Autodesk Inventor part; units mm, degrees
ref_plane "Work Plane1" through (-4.5785, -14.9902, 9) normal (0, 0, -1) x (0, 1, 0)
ref_plane "YZ Plane" through (0, 0, 0) normal (1, 0, 0) x (0, 1, 0)
ref_plane "XZ Plane" through (0, 0, 0) normal (0, 1, 0) x (-1, 0, 0)
sketch "Sketch1" plane through (0, 0, 0) normal (0, 0, 1) x (1, 0, 0)
  arc A0 (-8.6401, -8.1682) -> (6.2316, -10.1261) centre (-1.5676, -11.9073) ccw
  line L0 (7.4345, -0.9889) -> (6.2316, -10.1261)
  line L1 (-7.4371, 0.969) -> (7.4345, -0.9889)
  line L2 (-8.6401, -8.1682) -> (-7.4371, 0.969)
  line L3 (0.03, -17.852) -> (-0.1568, -19.2714)
  line L4 (-0.1568, -19.2714) -> (-0.6894, -19.2013)
  spline S0 degree 3 poles (-0.6894, -19.2013) (-0.7386, -19.1939) (-0.8276, -19.1805) (-0.9085, -19.1413) (-0.9446, -19.1238) knots 0 0 0 0 0.014823 0.02681 0.02681 0.02681 0.02681
  spline S1 degree 3 poles (-0.9446, -19.1238) (-0.9734, -19.1035) (-1.0308, -19.0631) (-1.0644, -19.0015) (-1.0811, -18.9709) knots 0 0 0 0 0.010419 0.020741 0.020741 0.020741 0.020741
  spline S2 degree 3 poles (-1.0811, -18.9709) (-1.0934, -18.9389) (-1.1175, -18.8762) (-1.1139, -18.8091) (-1.1121, -18.7762) knots 0 0 0 0 0.010155 0.019912 0.019912 0.019912 0.019912
  spline S3 degree 3 poles (-1.1121, -18.7762) (-1.106, -18.7465) (-1.0937, -18.6864) (-1.0581, -18.6365) (-1.0402, -18.6114) knots 0 0 0 0 0.008998 0.018167 0.018167 0.018167 0.018167
  spline S4 degree 3 poles (-1.0402, -18.6114) (-1.0175, -18.5881) (-0.9702, -18.5394) (-0.907, -18.5143) (-0.874, -18.5012) knots 0 0 0 0 0.009628 0.020138 0.020138 0.020138 0.020138
  spline S5 degree 3 poles (-0.874, -18.5012) (-0.912, -18.4819) (-0.9849, -18.4448) (-1.0323, -18.3782) (-1.055, -18.3464) knots 0 0 0 0 0.012589 0.024139 0.024139 0.024139 0.024139
  spline S6 degree 3 poles (-1.055, -18.3464) (-1.071, -18.3116) (-1.1036, -18.2405) (-1.0985, -18.1623) (-1.096, -18.1224) knots 0 0 0 0 0.011297 0.023097 0.023097 0.023097 0.023097
  spline S7 degree 3 poles (-1.096, -18.1224) (-1.09, -18.0901) (-1.0782, -18.0263) (-1.0456, -17.9702) (-1.0294, -17.9425) knots 0 0 0 0 0.009763 0.019307 0.019307 0.019307 0.019307
  spline S8 degree 3 poles (-1.0294, -17.9425) (-1.0117, -17.9179) (-0.9781, -17.8713) (-0.9305, -17.8392) (-0.9079, -17.824) knots 0 0 0 0 0.009007 0.017087 0.017087 0.017087 0.017087
  spline S9 degree 3 poles (-0.9079, -17.824) (-0.8832, -17.8123) (-0.8309, -17.7874) (-0.7736, -17.7788) (-0.7433, -17.7743) knots 0 0 0 0 0.008157 0.017283 0.017283 0.017283 0.017283
  spline S10 degree 3 poles (-0.7433, -17.7743) (-0.7078, -17.7719) (-0.6303, -17.7668) (-0.5531, -17.7758) (-0.5112, -17.7807) knots 0 0 0 0 0.010638 0.023262 0.023262 0.023262 0.023262
  line L5 (-0.5112, -17.7807) -> (0.03, -17.852)
  line L6 (-3.4981, -17.3875) -> (-3.685, -18.8069)
  line L7 (-3.685, -18.8069) -> (-3.8728, -18.7821)
  line L8 (-3.8728, -18.7821) -> (-3.7802, -18.0783)
  line L9 (-3.7802, -18.0783) -> (-4.5777, -18.6893)
  line L10 (-4.5777, -18.6893) -> (-4.8323, -18.6558)
  line L11 (-4.8323, -18.6558) -> (-4.1612, -18.1591)
  line L12 (-4.1612, -18.1591) -> (-4.6716, -17.233)
  line L13 (-4.6716, -17.233) -> (-4.4237, -17.2656)
  line L14 (-4.4237, -17.2656) -> (-4.0129, -18.0506)
  line L15 (-4.0129, -18.0506) -> (-3.7507, -17.8546)
  line L16 (-3.7507, -17.8546) -> (-3.686, -17.3627)
  line L17 (-3.686, -17.3627) -> (-3.4981, -17.3875)
  circle A1 centre (-5.3501, -2.3316) radius 1.25
  circle A2 centre (-0.3929, -2.9842) radius 1.25
  circle A3 centre (4.5643, -3.6369) radius 1.25
  line L18 (-1.8861, -17.5997) -> (-1.7118, -17.6227)
  line L19 (-1.7118, -17.6227) -> (-1.858, -18.7332)
  spline S11 degree 3 poles (-1.858, -18.7332) (-1.8315, -18.7156) (-1.7741, -18.6776) (-1.7111, -18.6498) (-1.6771, -18.6349) knots 0 0 0 0 0.009512 0.020621 0.020621 0.020621 0.020621
  spline S12 degree 3 poles (-1.6771, -18.6349) (-1.6428, -18.6208) (-1.579, -18.5947) (-1.5125, -18.5771) (-1.4818, -18.569) knots 0 0 0 0 0.011121 0.020634 0.020634 0.020634 0.020634
  line L20 (-1.4818, -18.569) -> (-1.5039, -18.7374)
  spline S13 degree 3 poles (-1.5039, -18.7374) (-1.5538, -18.755) (-1.6511, -18.7893) (-1.7387, -18.8438) (-1.7815, -18.8703) knots 0 0 0 0 0.015802 0.030852 0.030852 0.030852 0.030852
  spline S14 degree 3 poles (-1.7815, -18.8703) (-1.8184, -18.8967) (-1.8862, -18.945) (-1.9379, -19.0101) (-1.9614, -19.0397) knots 0 0 0 0 0.013536 0.024817 0.024817 0.024817 0.024817
  line L21 (-1.9614, -19.0397) -> (-2.0737, -19.0249)
  line L22 (-2.0737, -19.0249) -> (-1.8861, -17.5997)
  spline S15 degree 3 poles (-2.4246, -18.241) (-2.4356, -18.317) (-2.4555, -18.4539) (-2.5069, -18.5823) (-2.5297, -18.6393) knots 0 0 0 0 0.02295 0.041329 0.041329 0.041329 0.041329
  spline S16 degree 3 poles (-2.5297, -18.6393) (-2.5543, -18.6843) (-2.6009, -18.7695) (-2.6782, -18.8281) (-2.7148, -18.8558) knots 0 0 0 0 0.015169 0.02877 0.02877 0.02877 0.02877
  spline S17 degree 3 poles (-2.7148, -18.8558) (-2.7553, -18.8752) (-2.84, -18.9157) (-2.9339, -18.9088) (-2.9828, -18.9052) knots 0 0 0 0 0.013229 0.027677 0.027677 0.027677 0.027677
  spline S18 degree 3 poles (-2.9828, -18.9052) (-3.0189, -18.8989) (-3.0882, -18.8866) (-3.1483, -18.8503) (-3.1772, -18.8328) knots 0 0 0 0 0.010877 0.0209 0.0209 0.0209 0.0209
  spline S19 degree 3 poles (-3.1772, -18.8328) (-3.2025, -18.812) (-3.254, -18.7696) (-3.2859, -18.7111) (-3.3021, -18.6815) knots 0 0 0 0 0.009749 0.019786 0.019786 0.019786 0.019786
  spline S20 degree 3 poles (-3.3021, -18.6815) (-3.3159, -18.6476) (-3.3452, -18.5759) (-3.3564, -18.4992) (-3.3624, -18.4588) knots 0 0 0 0 0.010931 0.023145 0.023145 0.023145 0.023145
  spline S21 degree 3 poles (-3.3624, -18.4588) (-3.3653, -18.409) (-3.3719, -18.2955) (-3.358, -18.1825) (-3.3502, -18.1191) knots 0 0 0 0 0.014931 0.034052 0.034052 0.034052 0.034052
  spline S22 degree 3 poles (-3.3502, -18.1191) (-3.3392, -18.0436) (-3.3193, -17.9073) (-3.2684, -17.7795) (-3.2458, -17.7226) knots 0 0 0 0 0.022803 0.041126 0.041126 0.041126 0.041126
  spline S23 degree 3 poles (-3.2458, -17.7226) (-3.2213, -17.6776) (-3.1749, -17.5922) (-3.0976, -17.5334) (-3.0611, -17.5056) knots 0 0 0 0 0.015164 0.028785 0.028785 0.028785 0.028785
  spline S24 degree 3 poles (-3.0611, -17.5056) (-3.0205, -17.4861) (-2.9355, -17.4453) (-2.8413, -17.4522) (-2.792, -17.4558) knots 0 0 0 0 0.013268 0.02779 0.02779 0.02779 0.02779
  spline S25 degree 3 poles (-2.792, -17.4558) (-2.7285, -17.4698) (-2.6047, -17.4969) (-2.5269, -17.5968) (-2.489, -17.6454) knots 0 0 0 0 0.01885 0.036767 0.036767 0.036767 0.036767
  spline S26 degree 3 poles (-2.489, -17.6454) (-2.4583, -17.7269) (-2.386, -17.9186) (-2.4105, -18.1233) (-2.4246, -18.241) knots 0 0 0 0 0.025776 0.060673 0.060673 0.060673 0.060673
  arc A4 (-10.5788, -7.5715) -> (8.2587, -10.0515) centre (-1.5676, -11.9073) ccw
  line L23 (-10.5788, -7.5715) -> (-9.159, 3.213)
  line L24 (-9.159, 3.213) -> (9.6785, 0.733)
  line L25 (9.6785, 0.733) -> (8.2587, -10.0515)
  point P0 (0, 0)
  dimension "d0" = 2
ref_plane "Work Plane1" through (-4.5785, -14.9902, 9) normal (0, 0, -1) x (0, 1, 0)
extrude "Extrusion1" add sketch "Sketch1" along normal up to surface (9 mm away) contours L23 L24 L25 A4
sketch "Sketch2" plane through (9.6785, 0.733, 9) normal (0.1305, 0.9914, 0) x (0.9914, -0.1305, 0)
  line L0 (-17.5, 0) -> (-17.5, 9)
  line L1 (-1.5, 0) -> (-1.5, 9)
  line L2 (-17.5, 0) -> (-1.5, 0)
  line L3 (-1.5, 0) -> (-1.5, 9)
  line L4 (-1.5, 9) -> (-17.5, 9)
  line L5 (-17.5, 9) -> (-17.5, 0)
  point P0 (-9.5, 9)
  point P1 (-1.5, 0)
extrude "Extrusion2" cut sketch "Sketch2" against normal blind 10
properties part number "PotHolder"
CAD build for the part. Positions are in the model's coordinates, mm. A direction names the side the tool comes from. Coordinates: 2 decimals unless noted, no trailing zeros. Write each loop counter-clockwise with the first axis right and the second up, starting at its lowest first coordinate (ties: lowest second). Pieces come first, ordered by that corner, then holes. Notation, with made-up numbers: (-10, 85.25) -> (29, 85.25) arc R28 ccw to (29, 121.25) -> close; hole circle Ø11 at (-7, 25). An arc over 180 degrees is marked (long way). Return JSON: item names as keys, results as strings. Group by question number.
Q1. Cut at A-A, the plane y = -13.25. Give the cut face in (x, z).
Q2. Cut at B-B, the plane z = 7. Give the cut face in (x, y), then the cut area to 3 significant figures.
Q3. Cut at C-C, the plane y = -10.5. Give the cut face in (x, z).
Q4. Pull direction Y, two halves, no side cores. Call faces 1 (the face through (-8.315, -1.872, 4.563)), 2 (the face through (-8, -17, 0)), 3 (the face through (6.31, -9.52, 4.44)): released by +Y, released by -Y, zero draft, split by the parting line, or undercut.
Q5. Drill centre lines: line 1 (X direction, y = -16.5, z = 3); line 2 (X direction, y = 0, z = 6.75); line 3 (Y direction, x = -1.75, z = 2.75). Where is each one in solid material? Low to high.
Q6. Which spindle directions (+Z, -Z, +X, -X, +Y, -Y) get a long thin tool onto all of the face, cutting with end or side? Do faces 4 (the face through (7.548, -3.96, 4.563)), 5 (the face through (-8.426, 3.116, 4.437)), 6 (the face through (-8.56, -7.57, 4.44)). Say none if no direction does.
Q7. Cut at D-D, the plane x = -3.75. Give the cut face in (y, z).
Q8. Flat gauge pins, fed straight in: pin 1 (3 mm diameter, centred on y = -2.5, z = 7, fed in from +X); pin 2 (4 mm diameter, centred on x = -7, z = 6, fed in from +Y); pin 3 (5 mm diameter, centred on y = -17, z = 4, fed in from -X). Where does each tip first touch, or does it go through?
Returned:
{
 "1": {"outline": "(-11.48, 0) -> (-9.45, 0) -> (-9.45, 9) -> (-11.48, 9) -> close; (6.32, 0) -> (8.34, 0) -> (8.34, 9) -> (6.32, 9) -> close"},
 "2": {"outline": "(-10.58, -7.57) arc R10 ccw (long way) to (8.26, -10.05) -> (9.68, 0.73) -> (8.19, 0.93) -> (6.89, -8.99) -> (6.39, -8.92) -> (6.23, -10.13) arc R8 cw (long way) to (-8.64, -8.17) -> (-8.48, -6.96) -> (-8.98, -6.9) -> (-7.67, 3.02) -> (-9.16, 3.21) -> close", "area": "103 mm2"},
 "3": {"outline": "(-11.47, 0) -> (-9.44, 0) -> (-9.44, 9) -> (-11.47, 9) -> close; (6.31, 0) -> (8.33, 0) -> (8.33, 9) -> (6.31, 9) -> close"},
 "4": {"face 1": "undercut", "face 2": "zero draft", "face 3": "released by +Y"},
 "5": {"line 1": "x = -10.45 to -8.12, 4.98 to 7.32", "line 2": "x = -9.58 to -8.07, 8.07 to 9.58", "line 3": "y = -21.91 to -19.91"},
 "6": {"face 4": "+Z, -Z, +Y", "face 5": "+Z, -Z, +X, +Y", "face 6": "+Z, -Z"},
 "7": {"outline": "(-21.67, 0) -> (-19.6, 0) -> (-19.6, 9) -> (-21.67, 9) -> close"},
 "8": {"pin 1": "stops at x = 9.45", "pin 2": "stops at y = 3.19", "pin 3": "stops at x = -11.23"}
}
